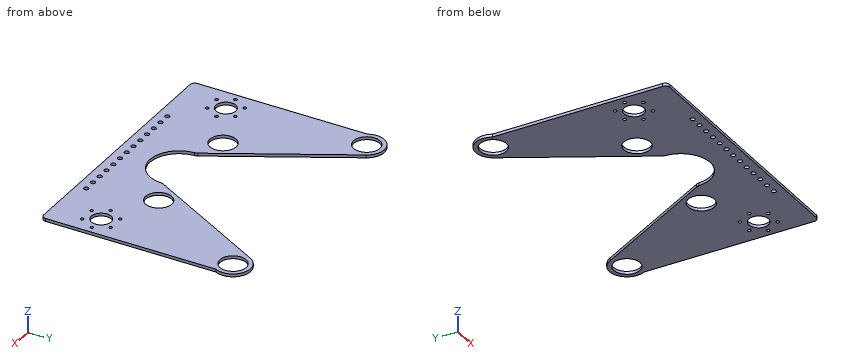
from build123d import *

# Parameters (mm, degrees)
SKETCH2_R           = 14.2875
SKETCH2_R_2         = 2.4892
SKETCH2_R_3         = 10.795
SKETCH2_R_4         = 1.778
BOSS_EXTRUDE1_DEPTH = 3.175
FILLET2_R           = 7.62


with BuildPart() as part:
    # Sketch2 → Boss-Extrude1 (new body)
    with BuildSketch(Plane.XY):
        with BuildLine():
            Line((142.632381685, 122.462939957), (142.632381685, -29.937060043))
            Line((142.632381685, -29.937060043), (142.632381685, -56.741928905))
            Line((142.632381685, -56.741928905), (142.632381685, -62.620500771))
            ThreePointArc((142.632381685, -62.620500771), (141.144484133, -66.21260322), (137.552381685, -67.700500771))
            Line((137.552381685, -67.700500771), (-137.552381685, -67.700500771))
            ThreePointArc((-137.552381685, -67.700500771), (-141.144484133, -66.21260322), (-142.632381685, -62.620500771))
            Line((-142.632381685, -62.620500771), (-142.632381685, -56.741928905))
            Line((-142.632381685, -56.741928905), (-142.632381685, -29.937060043))
            Line((-142.632381685, -29.937060043), (-142.632381685, 122.462939957))
            ThreePointArc((-142.632381685, 122.462939957), (-134.600001748, 148.101160684), (-108.918256202, 140.209048469))
            Line((-108.918256202, 140.209048469), (-31.75, 0))
            ThreePointArc((-31.75, 0), (0, -31.75), (31.75, 0))
            Line((31.75, 0), (108.918256202, 140.209048469))
            ThreePointArc((108.918256202, 140.209048469), (134.600001748, 148.101160684), (142.632381685, 122.462939957))
        make_face()
        with Locations((-60.484532313, 12.7)):
            Circle(SKETCH2_R, mode=Mode.SUBTRACT)
        with Locations((-125.726814921, 131.243846084)):
            Circle(SKETCH2_R, mode=Mode.SUBTRACT)
        with Locations((125.726814921, 131.243846084)):
            Circle(SKETCH2_R, mode=Mode.SUBTRACT)
        with Locations((60.484532313, 12.7)):
            Circle(SKETCH2_R, mode=Mode.SUBTRACT)
        with Locations((-76.5175, -57.15)):
            Circle(SKETCH2_R_2, mode=Mode.SUBTRACT)
        with Locations((-63.8175, -57.15)):
            Circle(SKETCH2_R_2, mode=Mode.SUBTRACT)
        with Locations((-51.1175, -57.15)):
            Circle(SKETCH2_R_2, mode=Mode.SUBTRACT)
        with Locations((-38.4175, -57.15)):
            Circle(SKETCH2_R_2, mode=Mode.SUBTRACT)
        with Locations((-25.7175, -57.15)):
            Circle(SKETCH2_R_2, mode=Mode.SUBTRACT)
        with Locations((-13.0175, -57.15)):
            Circle(SKETCH2_R_2, mode=Mode.SUBTRACT)
        with Locations((-0.3175, -57.15)):
            Circle(SKETCH2_R_2, mode=Mode.SUBTRACT)
        with Locations((12.3825, -57.15)):
            Circle(SKETCH2_R_2, mode=Mode.SUBTRACT)
        with Locations((25.0825, -57.15)):
            Circle(SKETCH2_R_2, mode=Mode.SUBTRACT)
        with Locations((37.7825, -57.15)):
            Circle(SKETCH2_R_2, mode=Mode.SUBTRACT)
        with Locations((50.4825, -57.15)):
            Circle(SKETCH2_R_2, mode=Mode.SUBTRACT)
        with Locations((63.1825, -57.15)):
            Circle(SKETCH2_R_2, mode=Mode.SUBTRACT)
        with Locations((75.8825, -57.15)):
            Circle(SKETCH2_R_2, mode=Mode.SUBTRACT)
        with Locations((-117.232381685, -16.900500771)):
            Circle(SKETCH2_R_3, mode=Mode.SUBTRACT)
        with Locations((117.232381685, -16.900500771)):
            Circle(SKETCH2_R_3, mode=Mode.SUBTRACT)
        with Locations((-135.012381685, -16.900500771)):
            Circle(SKETCH2_R_4, mode=Mode.SUBTRACT)
        with Locations((-126.122381685, -1.502569092)):
            Circle(SKETCH2_R_4, mode=Mode.SUBTRACT)
        with Locations((-108.342381685, -1.502569092)):
            Circle(SKETCH2_R_4, mode=Mode.SUBTRACT)
        with Locations((-99.452381685, -16.900500771)):
            Circle(SKETCH2_R_4, mode=Mode.SUBTRACT)
        with Locations((-108.342381685, -32.29843245)):
            Circle(SKETCH2_R_4, mode=Mode.SUBTRACT)
        with Locations((-126.122381685, -32.29843245)):
            Circle(SKETCH2_R_4, mode=Mode.SUBTRACT)
        with Locations((99.452381685, -16.900500771)):
            Circle(SKETCH2_R_4, mode=Mode.SUBTRACT)
        with Locations((108.342381685, -1.502569092)):
            Circle(SKETCH2_R_4, mode=Mode.SUBTRACT)
        with Locations((126.122381685, -1.502569092)):
            Circle(SKETCH2_R_4, mode=Mode.SUBTRACT)
        with Locations((135.012381685, -16.900500771)):
            Circle(SKETCH2_R_4, mode=Mode.SUBTRACT)
        with Locations((126.122381685, -32.29843245)):
            Circle(SKETCH2_R_4, mode=Mode.SUBTRACT)
        with Locations((108.342381685, -32.29843245)):
            Circle(SKETCH2_R_4, mode=Mode.SUBTRACT)
    extrude(amount=BOSS_EXTRUDE1_DEPTH)

    # Fillet2
    fillet2_edges = [part.edges().sort_by_distance(p)[0] for p in [
        (-31.75, 0, 1.5875),
        (31.75, 0, 1.5875),
    ]]
    fillet(fillet2_edges, radius=FILLET2_R)


solid = part.part
Verification items for the finished model (mm, model axes). Give positions to 0.01 mm unless a question says otherwise; leave off trailing zeros. Write each loop counter-clockwise with the first axis right and the second up, starting at its lowest first coordinate (ties: lowest second). Pieces come first, ordered by that corner, then holes. Notation, with made-up numbers: (29, -3) - (68, -3) arc R4 ccw to (68, 3) - close; hole circle Ø6 at (37, -12). An arc over 180 degrees is marked (long way). Answer as CSV lines item,"result". Start each with the question number.
1. Thickness scan on line 1 (X direction, y = 135.5, z = 2.4); line 2 (X direction, y = 5, z = 2.6); line 3 (Y direction, x = -62.5, z = 1.2). Record the ranges inside material, lowest first.
2. Sectioned sample at D-D (x = -93). Record the boundary of the cut face in (y, z) (1 decimal), then the cut area to 3 significant figures.
3. Sectioned sample at A-A (y = 12.7). Record the boundary of the cut face in (x, z) (3 decimals), then the cut area to 3 significant figures.
4. Depth check by flat-ended pin: pin 1 (5.5 mm diameter, centred on x = -25.72, y = -57.15, fed in from -Z); pin 2 (4.5 mm diameter, centred on x = 75.88, y = -57.15, fed in from -Z); pin 3 (1.5 mm diameter, centred on y = -11.5, z = 0.5, fed in from +X). Enter the tip coordinate at first touch or a pass-through.
5. Sectioned sample at C-C (z = 1.85). Count the separate pieces of the cut face and the enclosed holes in it, then the cut area to 3 significant figures.
6. Sectioned sample at B-B (x = 18.5). Record the boundary of the cut face in (y, z) (1 decimal).
Derived:
1,line 1,"-144.3 to -139.37, -112.09 to -106.33, 106.33 to 112.09, 139.37 to 144.3"
1,line 2,"-142.63 to -72.52, -48.45 to -34.5, 34.5 to 48.45, 72.52 to 142.63"
1,line 3,"-67.7 to -59.26, -55.04 to -1.44, 26.84 to 55.87"
2,outline,"(-67.7, 0) - (111.3, 0) - (111.3, 3.2) - (-67.7, 3.2) - close"
2,area,"568 mm²"
3,outline,"(-142.632, 0) - (-74.772, 0) - (-74.772, 3.175) - (-142.632, 3.175) - close; (-46.197, 0) - (-38.74, 0) - (-38.74, 3.175) - (-46.197, 3.175) - close; (38.74, 0) - (46.197, 0) - (46.197, 3.175) - (38.74, 3.175) - close; (74.772, 0) - (142.632, 0) - (142.632, 3.175) - (74.772, 3.175) - close"
3,area,"478 mm²"
4,pin 1,"z = 0"
4,pin 2,"through"
4,pin 3,"x = 142.63"
5,separate pieces,"1"
5,enclosed holes,"31"
5,area,"34,900 mm²"
6,outline,"(-67.7, 0) - (-25.8, 0) - (-25.8, 3.2) - (-67.7, 3.2) - close"
